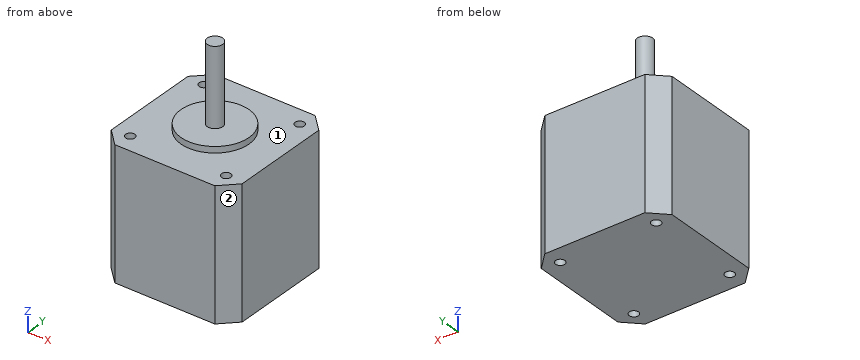
from build123d import *

# Parameters (mm, degrees)
F0_W     = 42.3
F0_H     = 42.3
F0_R     = 1.5
F1_DEPTH = 42
F2_R     = 11
F3_DEPTH = 2
F4_R     = 2.5
F5_DEPTH = 25
F6_SIZE  = 5


with BuildPart() as f1:
    # F0 (on Top) → F1 (new body)
    with BuildSketch(Plane.XY):
        Rectangle(F0_W, F0_H)
        with Locations((-15.5, -15.5)):
            Circle(F0_R, mode=Mode.SUBTRACT)
        with Locations((15.5, -15.5)):
            Circle(F0_R, mode=Mode.SUBTRACT)
        with Locations((-15.5, 15.5)):
            Circle(F0_R, mode=Mode.SUBTRACT)
        with Locations((15.5, 15.5)):
            Circle(F0_R, mode=Mode.SUBTRACT)
    extrude(amount=F1_DEPTH)

    # F2 (on face) → F3 (join)
    with BuildSketch(Plane.XY.offset(42)):
        Circle(F2_R)
    extrude(amount=F3_DEPTH)

    # F4 (on face) → F5 (join)
    with BuildSketch(Plane.XY.offset(44)):
        Circle(F4_R)
    extrude(amount=F5_DEPTH)

    # F6
    f6_edges = [f1.edges().sort_by_distance(p)[0] for p in [
        (-21.15, -21.15, 21),
        (21.15, -21.15, 21),
        (21.15, 21.15, 21),
        (-21.15, 21.15, 21),
    ]]
    chamfer(f6_edges, length=F6_SIZE)


solid = f1.part
Can you work these out from the model? Positions are in its coordinate system, mm. Face numbers are marked on the shaded views. A direction names the side the tool comes from. Coordinates: 2 decimals unless noted, no trailing zeros. Loops run counter-clockwise (first coordinate to the right, second up) from the corner with the lowest first, then second, coordinate; pieces in that order, holes last. Notation, with made-up numbers: M -11.5,-18.75 L 6.5,-18.75 A30 cw 6.5,17.25 Z; hole C 60,50.5 d1. An arc over 180 degrees is marked long. Return JSON: item names as keys, results as strings. Group by question number.
Item 1: On a 3-axis mill with a long thin cutter (end or side, diameter ignored), from which of +Z, -Z, +X, -X, +Y, -Y can I reach the whole of each face in a straight line? I mean the marked faces 1 and 2. Say none if no direction works.
Item 2: If I drill on L1, parallel to Y at x = 15.5, z = 22.5; L2, parallel to Y at x = 15, z = 14, over which ranges is the centre line in solid material (lowest first)? Write a range as from..to.
Item 3: I'm going to push flat-ended pins straight in: pin 1 Ø4 at (x, z) = (-2.5, 58) entering from -Y; pin 2 Ø2 at (x, y) = (-13, -7.5) entering from +Z. Where does each tip first touch, or does it pass through?
Item 4: Imagine slicing it at D-D (y = 12.5). Please give me the cut outline in (x, z), and give its area (3 significant figures).
Item 5: Imagine slicing it at B-B (x = 0.5). Please give me the cut outline in (y, z).
Item 6: Imagine slicing it at C-C (z = 61.5). Please give me the cut outline in (x, y).
Item 7: Imagine slicing it at A-A (y = 0). Please give me the cut outline in (x, z), and give its area (3 significant figures).
Verdict:
{
 "1": {"face 1": "+Z", "face 2": "+Z, -Z, +X, -Y"},
 "2": {"L1": "y = -21.15..-17, -14..14, 17..21.15", "L2": "y = -21.15..-16.91, -14.09..14.09, 16.91..21.15"},
 "3": {"pin 1": "stops at y = -2.45", "pin 2": "stops at z = 42"},
 "4": {"outline": "M -21.15,0 L 21.15,0 L 21.15,42 L -21.15,42 Z", "area": "1,780 mm^2"},
 "5": {"outline": "M -21.15,0 L 21.15,0 L 21.15,42 L 10.99,42 L 10.99,44 L 2.45,44 L 2.45,69 L -2.45,69 L -2.45,44 L -10.99,44 L -10.99,42 L -21.15,42 Z"},
 "6": {"outline": "C 0,0 d5"},
 "7": {"outline": "M -21.15,0 L 21.15,0 L 21.15,42 L 11,42 L 11,44 L 2.5,44 L 2.5,69 L -2.5,69 L -2.5,44 L -11,44 L -11,42 L -21.15,42 Z", "area": "1,950 mm^2"}
}
